Autodesk Inventor part; units mm, degrees
ref_plane "YZ Plane" through (0, 0, 0) normal (1, 0, 0) x (0, 1, 0)
ref_plane "XZ Plane" through (0, 0, 0) normal (0, 1, 0) x (-1, 0, 0)
ref_plane "XY Plane" through (0, 0, 0) normal (0, 0, 1) x (1, 0, 0)
sketch "Эскиз1" plane through (0, 0, 0) normal (0, 0, 1) x (1, 0, 0)
  line L0 (-63.5, -92) -> (-63.5, -81)
  line L1 (-63.5, -81) -> (-63.5, -92)
  line L2 (-75.5, -92) -> (-75.5, -80)
  line L3 (-96.5, -62) -> (-68.5, -62)
  line L4 (-68.5, -62) -> (-68.5, -52)
  line L5 (-68.5, -52) -> (-63.5, -52)
  line L6 (-63.5, -52) -> (-63.5, -76)
  line L7 (-63.5, -76) -> (-53.5, -76)
  line L8 (-53.5, -76) -> (-53.5, -81)
  line L9 (-63.5, -92) -> (-75.5, -92)
  line L10 (-53.5, -81) -> (-63.5, -81)
  line L11 (-96.5, -70) -> (-90.5, -70)
  line L12 (-90.5, -70) -> (-75.5, -80)
  line L13 (-96.5, -62) -> (-96.5, -70)
  line L14 (-115.8, 0) -> (19.3, 0)
  point P0 (0, 0)
  dimension "d0" = 12
  dimension "d1" = 5
  dimension "d2" = 10
  dimension "d3" = 30
  dimension "d5" = 12
  dimension "d7" = 10
  dimension "d8" = 6
  dimension "d9" = 5
  dimension "d10" = 8
  dimension "d11" = 21
  dimension "d13" = 70
revolve "Вращение1" add sketch "Эскиз1" angle 360 about axis through (-10, 0, 0) along (1, 0, 0)
chamfer "Фаска1" distance 2 angle 45 1 edges at (-96.5, 70, 0)
chamfer "Фаска2" distance 2 angle 45 1 edges at (-96.5, 62, 0)
chamfer "Фаска3" distance 2 angle 45 1 edges at (-53.5, 81, 0)
properties part number "2 крышка"
The listing builds one solid part. Answer for the finished solid, in the listing's coordinates (mm). A direction names the side the tool comes from. Give positions to 0.01 mm unless a question says otherwise; leave off trailing zeros. Loops run counter-clockwise (first coordinate to the right, second up) from the corner with the lowest first, then second, coordinate; pieces in that order, holes last. Notation, with made-up numbers: (4, -13.5) - (29, -13.5) arc R33 ccw to (29, 17.5) - close; hole circle Ø3 at (13, -36). An arc over 180 degrees is marked (long way). Return JSON: item names as keys, results as strings. Group by question number.
1. Determine the mould class of faces 1 (the conical face through (-53.625, -75.471, 23.767)), 2 (the flat face through (-68.5, 14.07, 50.23)), 3 (the flat face through (-96.5, 46, 45)) for opening direction Y: pulls with the +Y half, pulls with the -Y half, needs draft (parallel to the pull), parting line crosses it, or undercut.
2. Straight lines are drawn through the part: line 1 (Y direction, x = -66, z = 0); line 2 (Z direction, x = -60, y = 0). For each, find the intervals that lie inside material, in ascending order. Write a range as [from, to].
3. Find section C-C (x = -86). Write down the section's boundary in (y, z).
4. Which of the six approach directions +Z, -Z, +X, -X, +Y, -Y give full straight-line access (tool end or side, diameter ignored) to faces 4 (the flat face through (-75.5, 27.7, -75.4)), 5 (the cylindrical face through (-59.556, -43.545, 68.3)), 6 (the cylindrical face through (-69.584, 11.977, 91.217))?
5. Given pin 1 Ø2 at (x, z) = (-90, -56) entering from -Y; pin 2 Ø3 at (x, y) = (-63.5, 5.5) entering from -Z; pin 3 Ø8 at (y, z) = (-48.5, 56) entering from +X; pin 4 Ø12 at (y, z) = (72.5, 65) entering from +X, each flat-ended and moving along its own axis, determine where each tip first touches the part or whether it passes through.
Verdict:
{
 "1": {"face 1": "parting line crosses it", "face 2": "undercut", "face 3": "needs draft"},
 "2": {"line 1": "y = [-92, -52], [52, 92]", "line 2": "z = [-81, -76], [76, 81]"},
 "3": {"outline": "circle Ø146 at (0, 0); hole circle Ø124 at (0, 0)"},
 "4": {"face 4": "-X", "face 5": "+X", "face 6": "+X, -X"},
 "5": {"pin 1": "stops at y = -44.23", "pin 2": "stops at z = -91.91", "pin 3": "stops at x = -53.5", "pin 4": "stops at x = -63.5"}
}
